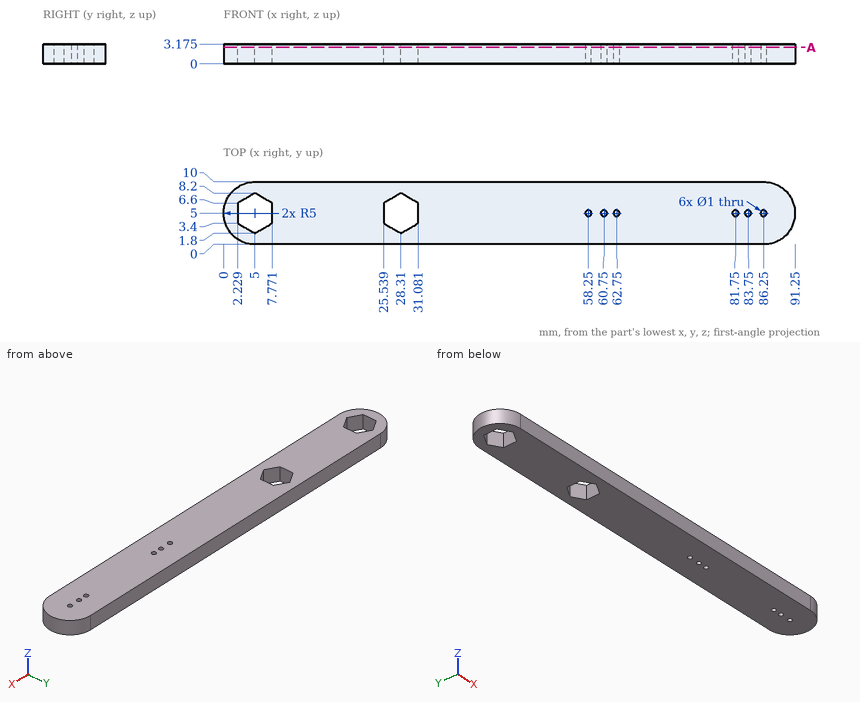
The figure shows three views and two pictorial views of one solid part (mm, origin at its lowest corner). Answer the questions. Round coordinates to 2 decimals unless told otherwise and drop trailing zeros.
Q1. Find the intervals of material crossed by line 1 along X through (y, z) = (2.5, 0.95); line 2 along Y through (x, z) = (60.75, 2.5); line 3 along Y through (x, z) = (86, 2.5), in increasing order.
Solution:
line 1: x = 0.67 to 3.79, 6.21 to 27.1, 29.52 to 90.58
line 2: y = 0 to 4.5, 5.5 to 10
line 3: y = 0 to 4.57, 5.43 to 10
Q2. Given pin 1 Ø1.5 at (y, z) = (8, 2) entering from -X (1 decimal); pin 2 Ø1 at (y, z) = (6, 2) entering from +X (3 decimals), each flat-ended and moving along its own axis, determine where each tip first touches the part or whether it passes through.
Solution:
pin 1: stops at x = 0.5
pin 2: stops at x = 91.225
Q3. A cutting plane is placed at A-A, the plane z = 2.65. Count the separate pieces of the cut face and the enclosed holes in it, then the cut area to 3 significant figures.
Solution:
separate pieces: 1
enclosed holes: 8
area: 833 mm2
